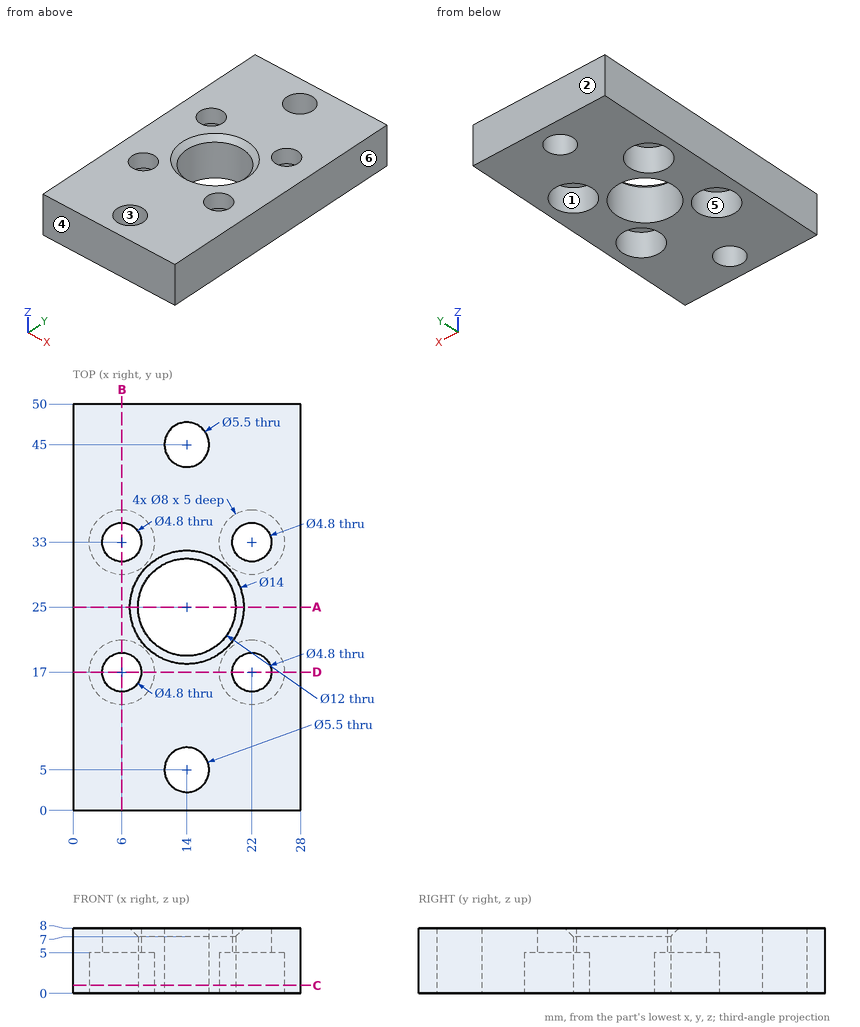
Could you check a few things on this drawing? It's one solid part, dimensions in mm from its lowest x, y, z. A direction names the side the tool comes from. Round coordinates to 2 decimals unless told otherwise and drop trailing zeros. Order: outer loops, then holes, each group sorted by start corner. A loop starts at its lowest first (then second) coordinate and runs counter-clockwise, first axis right, second up. Notation, with made-up numbers: (41, 8.25) -> (89, 8.25) arc R26 cw to (89, 27.25) -> close; hole circle Ø5 at (65.25, 69.5). An arc over 180 degrees is marked (long way). One line per question, with ' | ' between items.
Q1. If we section it at C-C on z = 1: Write out the boundary of the cut face in (x, y).
Computed values:
outline: (0, 0) -> (28, 0) -> (28, 50) -> (0, 50) -> close; hole circle Ø8 at (6, 17); hole circle Ø8 at (6, 33); hole circle Ø12 at (14, 25); hole circle Ø5.5 at (14, 5); hole circle Ø5.5 at (14, 45); hole circle Ø8 at (22, 17); hole circle Ø8 at (22, 33)
Q2. If we section it at A-A on y = 25: Write out the boundary of the cut face in (x, z).
Computed values:
outline: (0, 0) -> (8, 0) -> (8, 7) -> (7, 8) -> (0, 8) -> close; (20, 0) -> (28, 0) -> (28, 8) -> (21, 8) -> (20, 7) -> close
Q3. If I drill on line 1 (X direction, y = 17, z = 2.9); line 2 (X direction, y = 17, z = 6); line 3 (Y direction, x = 25, z = 4.5), over which ranges is the centre line in solid material (lowest first)? Write a range as from..to.
Computed values:
line 1: 0..2, 10..18, 26..28 | line 2: 0..3.6, 8.4..19.6, 24.4..28 | line 3: 0..14.35, 19.65..30.35, 35.65..50
Q4. If we section it at B-B on x = 6: Write out the boundary of the cut face in (y, z), plus the area to 3 significant figures.
Computed values:
outline: (0, 0) -> (13, 0) -> (13, 5) -> (14.6, 5) -> (14.6, 8) -> (0, 8) -> close; (19.4, 5) -> (21, 5) -> (21, 0) -> (29, 0) -> (29, 5) -> (30.6, 5) -> (30.6, 8) -> (19.4, 8) -> close; (35.4, 5) -> (37, 5) -> (37, 0) -> (50, 0) -> (50, 8) -> (35.4, 8) -> close | area: 291 mm²
Q5. I'm going to push flat-ended pins straight in: pin 1 (6 mm diameter, centred on x = 22, y = 17, fed in from -Z); pin 2 (4 mm diameter, centred on x = 6, y = 17, fed in from -Z). Where does each tip first touch, or does it pass through?
Computed values:
pin 1: z = 5 | pin 2: through
Q6. Which directions (+Z, -Z, +X, -X, +Y, -Y) give clear straight access to the entire face, cutting with the end or side of a thin tool? Please do the marked faces 1 and 2.
Computed values:
face 1: -Z | face 2: +Z, -Z, +X, -X, +Y
Q7. If we section it at D-D on y = 17: Write out the boundary of the cut face in (x, z).
Computed values:
outline: (0, 0) -> (2, 0) -> (2, 5) -> (3.6, 5) -> (3.6, 8) -> (0, 8) -> close; (8.4, 5) -> (10, 5) -> (10, 0) -> (18, 0) -> (18, 5) -> (19.6, 5) -> (19.6, 8) -> (8.4, 8) -> close; (24.4, 5) -> (26, 5) -> (26, 0) -> (28, 0) -> (28, 8) -> (24.4, 8) -> close
Q8. We'd pull the mould along Y, two halves only. Please class the marked faces 3, 4, 5 and 6: released by +Y, released by -Y, zero draft, split by the parting line, or undercut.
Computed values:
face 3: undercut | face 4: released by -Y | face 5: undercut | face 6: zero draft
